The model under review builds one solid part; all positions refer to its coordinate system, in mm. A direction names the side the tool comes from. Round coordinates to 2 decimals unless told otherwise and drop trailing zeros. Write each loop counter-clockwise with the first axis right and the second up, starting at its lowest first coordinate (ties: lowest second). Pieces come first, ordered by that corner, then holes. Notation, with made-up numbers: (47.25, 42.5) - (66.25, 42.5) arc R25 ccw to (66.25, 63.5) - close; hole circle Ø8 at (15, -3). An arc over 180 degrees is marked (long way). Write each question's results on one line, items separated by ' | '.
```python
from build123d import *
from OCP.BRepFilletAPI import BRepFilletAPI_MakeChamfer

# Parameters (mm, degrees)
SKETCH1_R           = 25.908
BOSS_EXTRUDE1_DEPTH = 15.875
BOSS_EXTRUDE1_DRAFT = -15
SKETCH2_R           = 25.4
BOSS_EXTRUDE2_DEPTH = 101.6
SKETCH5_R           = 22.86
CUT_EXTRUDE2_DEPTH  = 114.935
SKETCH6_R           = 20.32
CUT_EXTRUDE3_DEPTH  = 2.54
CHAMFER1_SIZE       = 0.762
CHAMFER1_SIZE2      = 0.622170395
CUT_EXTRUDE6_DEPTH  = 7.62


with BuildPart() as part:
    # Sketch1 → Boss-Extrude1 (with draft: the straight prism first)
    with BuildSketch(Plane(origin=(0, 0, 0), x_dir=(1, 0, 0), z_dir=(0, 1, 0))):
        Circle(SKETCH1_R)
    extrude(amount=BOSS_EXTRUDE1_DEPTH)
    # Boss-Extrude1: the draft: its side faces are tilted about the plane it starts from
    boss_extrude1_sides = [part.faces().sort_by_distance(p)[0] for p in [
        (-25.908, 7.9375, 0),
    ]]
    draft(boss_extrude1_sides, Plane(origin=(0, 0, 0), x_dir=(1, 0, 0), z_dir=(0, 1, 0)), BOSS_EXTRUDE1_DRAFT)

    # Sketch2 → Boss-Extrude2 (add)
    with BuildSketch(Plane(origin=(0, 15.875, 0), x_dir=(1, 0, 0), z_dir=(0, 1, 0))):
        with Locations(Location((0, 0, 0), (0, 0, 270))):
            Circle(SKETCH2_R)
    extrude(amount=BOSS_EXTRUDE2_DEPTH)

    # Sketch5 → Cut-Extrude2 (cut)
    with BuildSketch(Plane.XZ):
        with Locations(Location((0, 0, 0), (0, 0, 270))):
            Circle(SKETCH5_R)
    extrude(amount=-CUT_EXTRUDE2_DEPTH, mode=Mode.SUBTRACT)

    # Sketch6 → Cut-Extrude3 (cut)
    with BuildSketch(Plane(origin=(0, 117.475, 0), x_dir=(1, 0, 0), z_dir=(0, 1, 0))):
        with Locations(Location((0, 0, 0), (0, 0, 270))):
            Circle(SKETCH6_R)
    extrude(amount=-CUT_EXTRUDE3_DEPTH, mode=Mode.SUBTRACT)

    # Chamfer1: one chamfer whose edges measure the first distance from different faces: ONE call of the kernel's chamfer builder (chamfer() names one face for all edges)
    chamfer1_edges_1 = [part.edges().sort_by_distance(p)[0] for p in [
        (0, 117.475, -20.32),
        (0, 117.475, -25.4),
    ]]
    chamfer1_edges_2 = [part.edges().sort_by_distance(p)[0] for p in [
        (-30.16169343, 15.875, 0),
    ]]
    chamfer1_side_2 = [part.faces().sort_by_distance(p)[0] for p in [
        (-28.034846715, 7.9375, 0),
    ]]
    chamfer1 = BRepFilletAPI_MakeChamfer(part.part.solid().wrapped)
    for e in chamfer1_edges_1:
        chamfer1.Add(CHAMFER1_SIZE, e.wrapped)
    for e in chamfer1_edges_2:
        chamfer1.Add(CHAMFER1_SIZE, CHAMFER1_SIZE2, e.wrapped, chamfer1_side_2[0].wrapped)  # the first distance lies on this face
    add(Compound.cast(chamfer1.Shape()), mode=Mode.REPLACE)

    # Sketch7 → Cut-Extrude6 (cut)
    with BuildSketch(Plane(origin=(25.4, 0, 0), x_dir=(0, 0, -1), z_dir=(1, 0, 0))):
        with BuildLine():
            Line((-12.7, 87.63), (-12.7, 33.655))
            ThreePointArc((-12.7, 33.655), (0, 20.955), (12.7, 33.655))
            Line((12.7, 33.655), (12.7, 87.63))
            ThreePointArc((12.7, 87.63), (0, 100.33), (-12.7, 87.63))
        make_face()
    extrude(amount=-CUT_EXTRUDE6_DEPTH, mode=Mode.SUBTRACT)


solid = part.part
```
Q1. Tool access review of faces 1 (the flat face through (13, 15.875, -22)), 2 (the flat face through (-1.59, 114.935, 20.43)), 3 (the flat face through (11.1, 117.475, 18.1)), 4 (the flat face through (21, 61, 12.7)): name each direction out of +Z, -Z, +X, -X, +Y, -Y from which nothing blocks a thin tool from reaching the whole face with its end or side.
Evaluation:
face 1: +Y | face 2: -Y | face 3: +Z, -Z, +X, -X, +Y | face 4: +X
Q2. We need section A-A (z = 0). State the section outline as (x, y) points (3 decimals), plus the area to 3 significant figures.
Evaluation:
outline: (-29.964, 15.139) - (-25.908, 0) - (-22.86, 0) - (-22.86, 114.935) - (-20.32, 114.935) - (-20.32, 116.713) - (-21.082, 117.475) - (-24.638, 117.475) - (-25.4, 116.713) - (-25.4, 15.875) - (-29.54, 15.875) - close; (20.32, 114.935) - (22.86, 114.935) - (22.86, 100.33) - (25.4, 100.33) - (25.4, 116.713) - (24.638, 117.475) - (21.082, 117.475) - (20.32, 116.713) - close; (22.86, 0) - (25.908, 0) - (29.964, 15.139) - (29.54, 15.875) - (25.4, 15.875) - (25.4, 20.955) - (22.86, 20.955) - close | area: 490 mm^2
Q3. We need section D-D (y = 66). State the section outline as (x, z) points, plus the area to 3 significant figures.
Evaluation:
outline: (19.01, -12.7) arc R22.86 cw (long way) to (19.01, 12.7) - (22, 12.7) arc R25.4 ccw (long way) to (22, -12.7) - close | area: 317 mm^2
Q4. We need section C-C (y = 19). State the section outline as (x, z) points.
Evaluation:
outline: circle Ø50.8 at (0, 0); hole circle Ø45.72 at (0, 0)
Q5. The part is to be moulded in two halves that separate along Z. For faces 5 (the cylindrical face through (20.147, 115.836, -2.645)), 6 (the flat face through (2, 0, 23)), 7 (the cylindrical face through (23.671, 100.327, -0.279)), 8 (the cylindrical face through (-24.796, 65.588, -5.506)), say which applies: released by +Z, released by -Z, zero draft, split by the parting line, or undercut.
Evaluation:
face 5: undercut | face 6: zero draft | face 7: undercut | face 8: split by the parting line
Q6. We need section B-B (x = 0). State the section outline as (y, z) points (3 decimals), plus the area to 3 significant figures.
Evaluation:
outline: (0, -25.908) - (15.139, -29.964) - (15.875, -29.54) - (15.875, -25.4) - (116.713, -25.4) - (117.475, -24.638) - (117.475, -21.082) - (116.713, -20.32) - (114.935, -20.32) - (114.935, -22.86) - (0, -22.86) - close; (0, 22.86) - (114.935, 22.86) - (114.935, 20.32) - (116.713, 20.32) - (117.475, 21.082) - (117.475, 24.638) - (116.713, 25.4) - (15.875, 25.4) - (15.875, 29.54) - (15.139, 29.964) - (0, 25.908) - close | area: 692 mm^2
Q7. Insertion check: P1, Ø5, axis at y = 64, z = 21, coming from the -X side; P2, Ø1.5, axis at y = 59.5, z = 21, coming from the -X side; P3, Ø1, axis at x = 0, y = 102.5, coming from the -Z side; P4, Ø2, axis at x = -9.5, z = -16, coming from the -Y side. Each pin has a flat end and moves straight along its axis. Give the tip position at first contact, or say it passes through.
Evaluation:
P1: stops at x = -17.4 | P2: stops at x = -15.33 | P3: stops at z = -25.4 | P4: passes through
Q8. For probe 1 along X at (y, z) = (115, 0); probe 2 along X at (y, z) = (19, 15); probe 3 along Y at (x, z) = (-3, 25.5) (3 decimals), list the stretches that pass through material, from the lowest coordinate up.
Evaluation:
probe 1: x = -25.4 to -20.32, 20.32 to 25.4 | probe 2: x = -20.5 to -17.25, 17.25 to 20.5 | probe 3: y = 0 to 15.875
